from build123d import *

# Parameters (mm, degrees)
F1_DEPTH = 44
F2_R     = 4
F3_DEPTH = 25
F5_DEPTH = 25
F6_R     = 3
F7_R     = 10
F8_R     = 7.25
F9_DEPTH = 25


with BuildPart() as f1:
    # F0 (on Front) → F1 (new body)
    with BuildSketch(Plane.XZ):
        Polygon((0, 70), (0, 0), (3, 0), (3, 67), (33, 67), (33, 0), (36, 0), (36, 70), align=None)
    extrude(amount=F1_DEPTH)

    # F2 (on face) → F3 (cut)
    with BuildSketch(Plane.YZ.offset(36)):
        with Locations((-34, 10)):
            Circle(F2_R)
        Polygon((0, 0), (0, 70), (-22, 0), align=None)
    extrude(amount=-F3_DEPTH, mode=Mode.SUBTRACT)

    # F4 (on face) → F5 (cut)
    with BuildSketch(Plane(origin=(0, 0, 0), x_dir=(0, -1, 0), z_dir=(-1, 0, 0))):
        Polygon((22, 0), (0, 70), (0, 0), align=None)
        with BuildLine():
            Line((32.75, 15.6304840334), (32.75, 13.6304840334))
            ThreePointArc((32.75, 13.6304840334), (34, 6.1603497142), (35.25, 13.6304840334))
            Line((35.25, 13.6304840334), (35.25, 15.6304840334))
            Line((35.25, 15.6304840334), (32.75, 15.6304840334))
        make_face()
    extrude(amount=-F5_DEPTH, mode=Mode.SUBTRACT)

    # F6
    f6_edges = [f1.edges().sort_by_distance(p)[0] for p in [
        (33, -22.471429, 67),
        (3, -22.471429, 67),
        (36, -22, 70),
        (0, -22, 70),
    ]]
    fillet(f6_edges, radius=F6_R)

    # F7
    f7_edges = [f1.edges().sort_by_distance(p)[0] for p in [
        (1.5, -22, 0),
        (1.5, -44, 0),
        (34.5, -44, 0),
        (34.5, -22, 0),
    ]]
    fillet(f7_edges, radius=F7_R)

    # F8 (on face) → F9 (cut)
    with BuildSketch(Plane.XY.offset(70)):
        with Locations((18, -22)):
            Circle(F8_R)
    extrude(amount=-F9_DEPTH, mode=Mode.SUBTRACT)


solid = f1.part
The model under review builds one solid part; all positions refer to its coordinate system, in mm. A direction names the side the tool comes from. Coordinates: 2 decimals unless noted, no trailing zeros. Loops run counter-clockwise (first coordinate to the right, second up) from the corner with the lowest first, then second, coordinate; pieces in that order, holes last.
(1) Wall thickness on L1, parallel to X at y = -25.5, z = 54.5; L2, parallel to Y at x = 32, z = 67; L3, parallel to Z at x = 19.5, y = -33: over which ranges is each line inside the solid? List them lowest first.
Determined:
L1: x = 0 to 3, 33 to 36
L2: y = -44 to -0.94
L3: z = 67 to 70
(2) Insertion check: P1, Ø5, axis at y = -34, z = 10, coming from the +X side; P2, Ø3, axis at x = 32, z = 58.5, coming from the +Y side; P3, Ø0.6, axis at x = 1, z = 14, coming from the +Y side. Each pin has a flat end and moves straight along its axis. Give the tip position at first contact, or say it passes through.
Determined:
P1: passes through
P2: stops at y = -3.26
P3: stops at y = -17.51
(3) Tool access review of faces 1 (the flat face through (33, -27, 40)), 2 (the cylindrical face through (21.9, -15.89, 68.52)), 3 (the cylindrical face through (35, -38, 10)): name each direction out of +Z, -Z, +X, -X, +Y, -Y from which nothing blocks a thin tool from reaching the whole face with its end or side.
Determined:
face 1: -Z, +Y, -Y
face 2: +Z, -Z
face 3: +X
(4) Consider section A-A, the plane x = 18. Give the boundary of the cut face in (y, z).
Determined:
outline: (-44, 67) - (-29.25, 67) - (-29.25, 70) - (-44, 70) - close; (-14.75, 67) - (-0.94, 67) - (0, 70) - (-14.75, 70) - close
(5) Consider section D-D, the plane x = 12.5. Give the boundary of the cut face in (y, z).
Determined:
outline: (-44, 67) - (-26.72, 67) - (-26.72, 70) - (-44, 70) - close; (-17.28, 67) - (-0.94, 67) - (0, 70) - (-17.28, 70) - close
(6) Consider section B-B, the plane y = -22. Give the boundary of the cut face in (x, z).
Determined:
outline: (0, 3.21) - (3, 3.21) - (3, 64) arc R3 cw to (6, 67) - (10.75, 67) - (10.75, 70) - (3, 70) arc R3 ccw to (0, 67) - close; (25.25, 67) - (30, 67) arc R3 cw to (33, 64) - (33, 3.21) - (36, 3.21) - (36, 67) arc R3 ccw to (33, 70) - (25.25, 70) - close
(7) Draft analysis for pull direction X (two halves, no side actions). For faces 4 (the cylindrical face through (0.86, -22.31, 69.1)), 5 (the flat face through (12, -27, 67)), 6 (the flat face through (25, -17, 70)), 7 (the flat face through (3, -27, 39)), state which applies: +X half, -X half, draft (parallel to the pull), parting line (faces both ways), or undercut.
Determined:
face 4: -X half
face 5: undercut
face 6: draft
face 7: undercut
(8) Consider section C-C, the plane y = -11.5. Give the boundary of the cut face in (x, z).
Determined:
outline: (0, 33.41) - (3, 33.41) - (3, 64) arc R3 cw to (6, 67) - (30, 67) arc R3 cw to (33, 64) - (33, 33.41) - (36, 33.41) - (36, 67) arc R3 ccw to (33, 70) - (3, 70) arc R3 ccw to (0, 67) - close
